Here's the drawing with two shaded views (mm, measured from the low corner). I have some questions. Coordinates: 2 decimals unless noted, no trailing zeros. Write each loop counter-clockwise with the first axis right and the second up, starting at its lowest first coordinate (ties: lowest second). Pieces come first, ordered by that corner, then holes.
Item 1: If we section it at A-A (z = 3.25): Count the separate pieces of the cut face and the enclosed holes in it, then the cut area to 3 significant figures.
Item 2: If we section it at B-B (y = 15.5): Please give me the cut outline in (x, z).
Item 3: I'm going to push flat-ended pins straight in: pin 1 Ø3 at (x, y) = (79.5, 16) entering from -Z; pin 2 Ø2 at (y, z) = (63.5, 4.5) entering from -X. Where does each tip first touch, or does it pass through?
Item 4: If we section it at C-C (x = 12): Please give me the cut outline in (y, z), then the cut area to 3 significant figures.
Item 5: If I drill on line 1 (Z direction, x = 10, y = 55), over which ranges is the centre line in solid material (lowest first)?
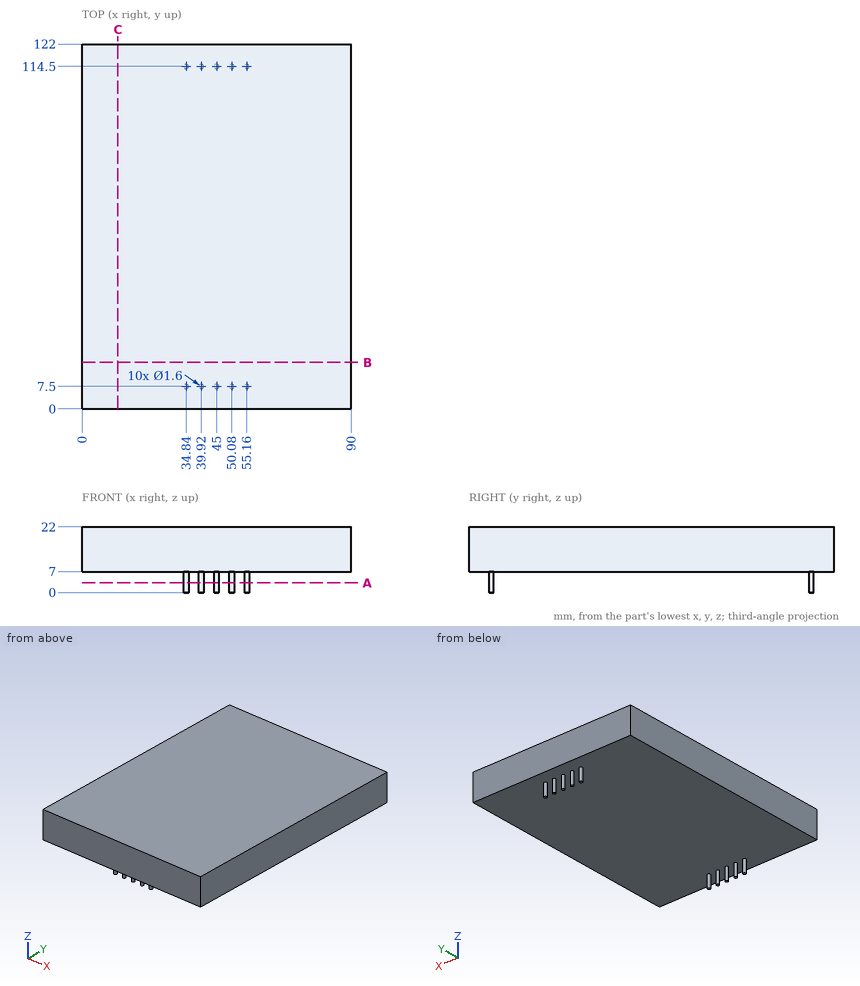
Answer list:
1. separate pieces: 10
1. enclosed holes: 0
1. area: 20.1 mm2
2. outline: (0, 7) - (90, 7) - (90, 22) - (0, 22) - close
3. pin 1: stops at z = 7
3. pin 2: passes through
4. outline: (0, 7) - (122, 7) - (122, 22) - (0, 22) - close
4. area: 1,830 mm2
5. line 1: z = 7 to 22
